```python
from build123d import *
from build123d.topology import SkipClean

# Parameters (mm, degrees)
SKETCH1_R               = 2.5
BOSS_EXTRUDE1_DEPTH     = 5
SKETCH2_R               = 1.25
CUT_EXTRUDE1_DEPTH      = 10
BOSS_EXTRUDE2_START     = 0.1
SKETCH4_R               = 2.5
SKETCH4_R_2             = 2.107798696
BOSS_EXTRUDE2_DEPTH     = 0.1
SKETCH5_R               = 2.5
SKETCH5_R_2             = 2.269592882
BOSS_EXTRUDE3_DEPTH     = 0.1
BOSS_EXTRUDE5_START     = -0.098685172
BOSS_EXTRUDE5_DEPTH     = 5.286540914
SKETCH12_W              = 5.286540914
SKETCH12_H              = 2.95536745
BOSS_EXTRUDE6_DEPTH     = 30
BOSS_EXTRUDE7_START     = -5.286541
SKETCH13_R              = 5
BOSS_EXTRUDE7_DEPTH     = 5.286541
CUT_EXTRUDE2_DEPTH      = 56.479378316
CUT_EXTRUDE2_DEPTH_BACK = 56.479378316
SKETCH14_R              = 2.5


# Read off the part's stored shape, not the designer's step: Boss-Extrude5
with BuildPart() as part:
    # Sketch1 → Boss-Extrude1 (new body)
    with BuildSketch(Plane(origin=(0, 0, 0), x_dir=(0, 0, -1), z_dir=(1, 0, 0))):
        Circle(SKETCH1_R)
    extrude(amount=BOSS_EXTRUDE1_DEPTH)

    # Sketch2 → Cut-Extrude1 (cut)
    with BuildSketch(Plane.ZY):
        Circle(SKETCH2_R)
    extrude(amount=-CUT_EXTRUDE1_DEPTH, mode=Mode.SUBTRACT)

    # Sketch4 → Boss-Extrude2 (add)
    with BuildSketch(Plane.ZY.offset(BOSS_EXTRUDE2_START)):
        Circle(SKETCH4_R)
        Circle(SKETCH4_R_2, mode=Mode.SUBTRACT)
    extrude(amount=-BOSS_EXTRUDE2_DEPTH)

    # Sketch5 → Boss-Extrude3 (add)
    with BuildSketch(Plane(origin=(5, 0, 0), x_dir=(0, 0, -1), z_dir=(1, 0, 0))):
        with Locations(Location((0, 0, 0), (0, 0, 180))):
            Circle(SKETCH5_R)
        Circle(SKETCH5_R_2, mode=Mode.SUBTRACT)
    extrude(amount=BOSS_EXTRUDE3_DEPTH)

    # Boss-Extrude5 outline → Boss-Extrude5 (add)
    with SkipClean():  # the faces are left unmerged after this step: merging them gives an invalid solid
        with BuildSketch(Plane.YZ.offset(BOSS_EXTRUDE5_START)):
            with BuildLine():
                Line((-1.477683725, 20), (-1.477683725, 2.016544274))
                ThreePointArc((-1.477683725, 2.016544274), (0, 2.5), (1.477683725, 2.016544274))
                Line((1.477683725, 2.016544274), (1.477683725, 20))
                Line((1.477683725, 20), (-1.477683725, 20))
            make_face()
        extrude(amount=BOSS_EXTRUDE5_DEPTH)

    # Sketch12 → Boss-Extrude6 (add)
    with SkipClean():  # the faces are left unmerged after this step: merging them gives an invalid solid
        with BuildSketch(Plane.XY.offset(20)):
            with Locations((2.544585285, 0)):
                Rectangle(SKETCH12_W, SKETCH12_H)
        extrude(amount=BOSS_EXTRUDE6_DEPTH)

    # Sketch13 → Boss-Extrude7 (add)
    with SkipClean():  # the faces are left unmerged after this step: merging them gives an invalid solid
        with BuildSketch(Plane(origin=(5.187855742, 0, 0), x_dir=(0, 0, -1), z_dir=(1, 0, 0)).offset(BOSS_EXTRUDE7_START)):
            with Locations((-50, 0)):
                Circle(SKETCH13_R)
        extrude(amount=BOSS_EXTRUDE7_DEPTH)

    # Sketch14 → Cut-Extrude2 (cut, two sides: drawn at the far end of the back side and taken through both)
    with SkipClean():  # the faces are left unmerged after this step: merging them gives an invalid solid
        with BuildSketch(Plane(origin=(5.187855742, 0, 0), x_dir=(0, 0, -1), z_dir=(1, 0, 0)).offset(-CUT_EXTRUDE2_DEPTH_BACK)):
            with Locations((-50, 0)):
                Circle(SKETCH14_R)
        extrude(amount=CUT_EXTRUDE2_DEPTH + CUT_EXTRUDE2_DEPTH_BACK, mode=Mode.SUBTRACT)


solid = part.part
```
Read the model definition and answer for the solid it produces. Units are mm, in the model's axes. A direction names the side the tool comes from. Give positions to 0.01 mm unless a question says otherwise; leave off trailing zeros. Write each loop counter-clockwise with the first axis right and the second up, starting at its lowest first coordinate (ties: lowest second). Pieces come first, ordered by that corner, then holes. Notation, with made-up numbers: M -30.5,-19.75 L -17.5,-19.75 A37 ccw -17.5,16.25 Z; hole C 78,69.5 d5. An arc over 180 degrees is marked long. Put each result on its own line as item: value. Start each with the question number.
1. Consider line 1 along Y through (x, z) = (3.3, 50); line 2 along Y through (x, z) = (3.2, 0); line 3 along X through (y, z) = (0.25, 7.5). Determine where each line is inside the solid, lowest interval first.
2. The part is cut by section D-D, the plane y = 3.25. Give the vertices of the cut face in (x, z), and give its area (3 significant figures).
3. Each of these flat-tipped pins is pushed along its axis until it touches: pin 1 Ø3 at (x, y) = (1.5, 0.5) entering from +Z; pin 2 Ø1.6 at (x, z) = (1, 19.5) entering from +Y; pin 3 Ø2.5 at (y, z) = (0.5, -0.5) entering from +X; pin 4 Ø1.6 at (x, z) = (2, 30.5) entering from -Y. Where does it stop, or does it pass through?
4. Which of the six approach directions +Z, -Z, +X, -X, +Y, -Y give full straight-line access (tool end or side, diameter ignored) to faces 1 (the flat face through (0, -1, -1)), 2 (the cylindrical face through (3, 0, 55)), 3 (the flat face through (5, -1, -1)), 4 (the flat face through (3, -1.478, 23))?
5. The part is cut by section C-C, the plane z = 50. Give the vertices of the cut face in (x, y), and give its area (3 significant figures).
6. The part is cut by section B-B, the plane x = 2. Give the vertices of the cut face in (y, z).
7. For a pull along Z with two mould halves and no side action, classify faces 5 (the flat face through (-0.099, 0, 34)), 6 (the flat face through (3, 1.478, 23)) as released by +Z, released by -Z, zero draft, split by the parting line, or undercut.
8. The part is cut by section A-A, the plane z = 0. Give the vertices of the cut face in (x, y), and give its area (3 significant figures).
Final values:
1. line 1: y = -5 to -2.5, 2.5 to 5
1. line 2: y = -2.5 to -1.25, 1.25 to 2.5
1. line 3: x = -0.1 to 5.19
2. outline: M -0.1,46.2 L 5.19,46.2 L 5.19,53.8 L -0.1,53.8 Z
2. area: 40.2 mm²
3. pin 1: stops at z = 55
3. pin 2: stops at y = 1.48
3. pin 3: stops at x = 5
3. pin 4: stops at y = -1.48
4. face 1: -X
4. face 2: +X, -X
4. face 3: +X
4. face 4: +X, -X, -Y
5. outline: M -0.1,-5 L 5.19,-5 L 5.19,-2.5 L -0.1,-2.5 Z; M -0.1,2.5 L 5.19,2.5 L 5.19,5 L -0.1,5 Z
5. area: 26.4 mm²
6. outline: M -1.48,2.02 A2.5 ccw long 1.48,2.02 L 1.48,45.22 A5 ccw long -1.48,45.22 Z; hole C 0,50 d5; hole C 0,0 d2.5
7. face 5: zero draft
7. face 6: undercut
8. outline: M -0.1,-2.5 L 5.1,-2.5 L 5.1,-2.27 L 5,-2.27 L 5,-1.25 L 0,-1.25 L 0,-2.11 L -0.1,-2.11 Z; M -0.1,2.11 L 0,2.11 L 0,1.25 L 5,1.25 L 5,2.27 L 5.1,2.27 L 5.1,2.5 L -0.1,2.5 Z
8. area: 12.6 mm²
